from build123d import *

# Parameters (mm, degrees)
SKETCH1_W                                  = 300
SKETCH1_H                                  = 300
BOSS_EXTRUDE1_DEPTH                        = 5
CUT_EXTRUDE1_REACH                         = 214.191
SKETCH2_R                                  = 2.05
MIRROR1_AT_THE_SECOND_PLANE_COPY_1_REACH   = 214.191
MIRROR1_AT_THE_SECOND_PLANE_COPY_1_SKETC_R = 2.05
CUT_EXTRUDE2_REACH                         = 214.191
SKETCH3_W                                  = 80
SKETCH3_H                                  = 260
CUT_EXTRUDE3_REACH                         = 214.191
SKETCH4_R                                  = 2.05


with BuildPart() as part:
    # Sketch1 → Boss-Extrude1 (new body)
    with BuildSketch(Plane(origin=(0, 0, 0), x_dir=(1, 0, 0), z_dir=(0, 1, 0))):
        Rectangle(SKETCH1_W, SKETCH1_H)
    extrude(amount=BOSS_EXTRUDE1_DEPTH)

    # Sketch2 → Cut-Extrude1 (cut, up to next)
    with BuildSketch(Plane(origin=(0, 5, 0), x_dir=(1, 0, 0), z_dir=(0, 1, 0)), mode=Mode.PRIVATE) as cut_extrude1_sk1:
        with Locations(Location((-146, 146, 0), (0, 0, 270))):
            Circle(SKETCH2_R)
    cut_extrude1_tool1 = extrude(cut_extrude1_sk1.sketch, amount=-CUT_EXTRUDE1_REACH, mode=Mode.PRIVATE) & part.part
    cut_extrude1 = cut_extrude1_tool1.solids().sort_by_distance((-146, 5, -146))[0]
    add(cut_extrude1, mode=Mode.SUBTRACT)

    # Mirror1: Cut-Extrude1 across plane
    add(cut_extrude1.mirror(Plane(origin=(0, 0, 0), x_dir=(0, 0, 1), z_dir=(1, 0, 0))), mode=Mode.SUBTRACT)

    # Mirror1 at the second plane: Cut-Extrude1 across plane
    add(cut_extrude1.mirror(Plane.XY), mode=Mode.SUBTRACT)

    # Mirror1 at the second plane copy 1 sketc → Mirror1 at the second plane copy 1 (cut, up to next)
    with BuildSketch(Plane(origin=(0, 5, 0), x_dir=(-1, 0, 0), z_dir=(0, 1, 0)), mode=Mode.PRIVATE) as mirror1_at_the_second_plane_copy_1_sk1:
        with Locations(Location((-146, 146, 0), (0, 0, 270))):
            Circle(MIRROR1_AT_THE_SECOND_PLANE_COPY_1_SKETC_R)
    mirror1_at_the_second_plane_copy_1_tool1 = extrude(mirror1_at_the_second_plane_copy_1_sk1.sketch, amount=-MIRROR1_AT_THE_SECOND_PLANE_COPY_1_REACH, mode=Mode.PRIVATE) & part.part
    add(mirror1_at_the_second_plane_copy_1_tool1.solids().sort_by_distance((146, 5, 146))[0], mode=Mode.SUBTRACT)

    # Sketch3 → Cut-Extrude2 (cut, up to next)
    with BuildSketch(Plane(origin=(0, 5, 0), x_dir=(1, 0, 0), z_dir=(0, 1, 0)), mode=Mode.PRIVATE) as cut_extrude2_sk1:
        Rectangle(SKETCH3_W, SKETCH3_H)
    cut_extrude2_tool1 = extrude(cut_extrude2_sk1.sketch, amount=-CUT_EXTRUDE2_REACH, mode=Mode.PRIVATE) & part.part
    add(cut_extrude2_tool1.solids().sort_by_distance((0, 5, 0))[0], mode=Mode.SUBTRACT)

    # Sketch4 → Cut-Extrude3 (cut, up to next)
    with BuildSketch(Plane(origin=(0, 5, 0), x_dir=(1, 0, 0), z_dir=(0, 1, 0)), mode=Mode.PRIVATE) as cut_extrude3_sk1:
        with Locations(Location((-111, 36.46851285, 0), (0, 0, 270))):
            Circle(SKETCH4_R)
    cut_extrude3_tool1 = extrude(cut_extrude3_sk1.sketch, amount=-CUT_EXTRUDE3_REACH, mode=Mode.PRIVATE) & part.part
    # Sketch4 → Cut-Extrude3 (cut, up to next)
    with BuildSketch(Plane(origin=(0, 5, 0), x_dir=(1, 0, 0), z_dir=(0, 1, 0)), mode=Mode.PRIVATE) as cut_extrude3_sk2:
        with Locations(Location((-44, 36.46851285, 0), (0, 0, 270))):
            Circle(SKETCH4_R)
    cut_extrude3_tool2 = extrude(cut_extrude3_sk2.sketch, amount=-CUT_EXTRUDE3_REACH, mode=Mode.PRIVATE) & part.part
    # Sketch4 → Cut-Extrude3 (cut, up to next)
    with BuildSketch(Plane(origin=(0, 5, 0), x_dir=(1, 0, 0), z_dir=(0, 1, 0)), mode=Mode.PRIVATE) as cut_extrude3_sk3:
        with Locations(Location((-44, -31.53148715, 0), (0, 0, 270))):
            Circle(SKETCH4_R)
    cut_extrude3_tool3 = extrude(cut_extrude3_sk3.sketch, amount=-CUT_EXTRUDE3_REACH, mode=Mode.PRIVATE) & part.part
    # Sketch4 → Cut-Extrude3 (cut, up to next)
    with BuildSketch(Plane(origin=(0, 5, 0), x_dir=(1, 0, 0), z_dir=(0, 1, 0)), mode=Mode.PRIVATE) as cut_extrude3_sk4:
        with Locations(Location((-111, -31.53148715, 0), (0, 0, 270))):
            Circle(SKETCH4_R)
    cut_extrude3_tool4 = extrude(cut_extrude3_sk4.sketch, amount=-CUT_EXTRUDE3_REACH, mode=Mode.PRIVATE) & part.part
    cut_extrude3_1 = cut_extrude3_tool1.solids().sort_by_distance((-111, 5, -36.468513))[0]
    add(cut_extrude3_1, mode=Mode.SUBTRACT)
    cut_extrude3_2 = cut_extrude3_tool2.solids().sort_by_distance((-44, 5, -36.468513))[0]
    add(cut_extrude3_2, mode=Mode.SUBTRACT)
    cut_extrude3_3 = cut_extrude3_tool3.solids().sort_by_distance((-44, 5, 31.531487))[0]
    add(cut_extrude3_3, mode=Mode.SUBTRACT)
    cut_extrude3_4 = cut_extrude3_tool4.solids().sort_by_distance((-111, 5, 31.531487))[0]
    add(cut_extrude3_4, mode=Mode.SUBTRACT)
    cut_extrude3 = cut_extrude3_1 + cut_extrude3_2 + cut_extrude3_3 + cut_extrude3_4  # Cut-Extrude3 as one shape, for the pattern or mirror that repeats it

    # Mirror2: Cut-Extrude3 across plane
    add(cut_extrude3.mirror(Plane(origin=(0, 0, 0), x_dir=(0, 0, 1), z_dir=(1, 0, 0))), mode=Mode.SUBTRACT)


solid = part.part
For this review, take the finished solid that the model builds, in its own axes (mm). Round coordinates to 2 decimals unless told otherwise and drop trailing zeros. Order: outer loops, then holes, each group sorted by start corner. A loop starts at its lowest first (then second) coordinate and runs counter-clockwise, first axis right, second up. Notation, with made-up numbers: M 47,24.25 L 62,24.25 A26 cw 62,38.25 Z; hole C 11.5,25.5 d10. An arc over 180 degrees is marked long. Write each question's results on one line, items separated by ' | '. Start each with the question number.
1. Add section A-A (z = 70). State the section outline as (x, y) points, then the cut area to 3 significant figures.
2. Clearance check with a flat-ended pin moving along its axis: pin 1 Ø2.5 at (x, z) = (111, 31.53) entering from +Y. State where the tip first meets the part, or that it passes through.
3. To check wall thickness, follow L1, parallel to Z at x = -111.5, y = 2.45; L2, parallel to Z at x = -146, y = 3; L3, parallel to X at y = 3.8, z = -81. State the ranges of each line that lie inside material, in increasing order. Write a range as [from, to].
4. Add section B-B (x = 20). State the section outline as (y, z) points.
5. Add section C-C (y = 4.05). State how many separate pieces and enclosed holes the cut face has, then the cut area to 3 significant figures.
Output values:
1) outline: M -150,0 L -40,0 L -40,5 L -150,5 Z; M 40,0 L 150,0 L 150,5 L 40,5 Z | area: 1,100 mm^2
2) pin 1: through
3) L1: [-150, -38.46], [-34.48, 29.54], [33.52, 150] | L2: [-150, -148.05], [-143.95, 143.95], [148.05, 150] | L3: [-150, -40], [40, 150]
4) outline: M 0,-150 L 5,-150 L 5,-130 L 0,-130 Z; M 0,130 L 5,130 L 5,150 L 0,150 Z
5) separate pieces: 1 | enclosed holes: 13 | area: 69,000 mm^2
